Can you work these out from the drawing? Everything is in mm from the part's minimum corner. Give positions to 0.01 mm unless a question says otherwise; leave off trailing zeros. Write each loop counter-clockwise with the first axis right and the second up, starting at its lowest first coordinate (ties: lowest second). Pieces come first, ordered by that corner, then holes. Notation, with made-up numbers: (23, 18.5) - (74, 18.5) arc R17 cw to (74, 47.5) - close; hole circle Ø2 at (-17.5, 21). An arc over 180 degrees is marked (long way). Write each question's results on one line, items separated by ' | '. Start each with the question number.
Item 1: Suppose I cut it at D-D on x = 2.5. List the corners of the cut face in (y, z) for me, then the cut area to 3 significant figures.
Item 2: Please list where these lines run through material, in increasing order: line 1 along Y through (x, z) = (14.5, 14.25); line 2 along Y through (x, z) = (11.75, 12.25); line 3 along X through (y, z) = (20, 10.25).
Item 3: Will this pin go through, and if not, where does the flat tip stop? P1, Ø5, axis at x = 10, z = 9, coming from the -Y side.
Item 4: Suppose I cut it at C-C on z = 23.75. List the corners of the cut face in (x, y) for me, then the cut area to 3 significant figures.
Item 5: We'd pull the mould along Y, two halves only. Please class the marked faces 1, 2 and 3: +Y half, -Y half, draft (parallel to the pull), parting line (faces both ways), or undercut.
Item 6: Suppose I cut it at A-A on y = 14.5. List the corners of the cut face in (x, z) for me, then the cut area to 4 significant figures.
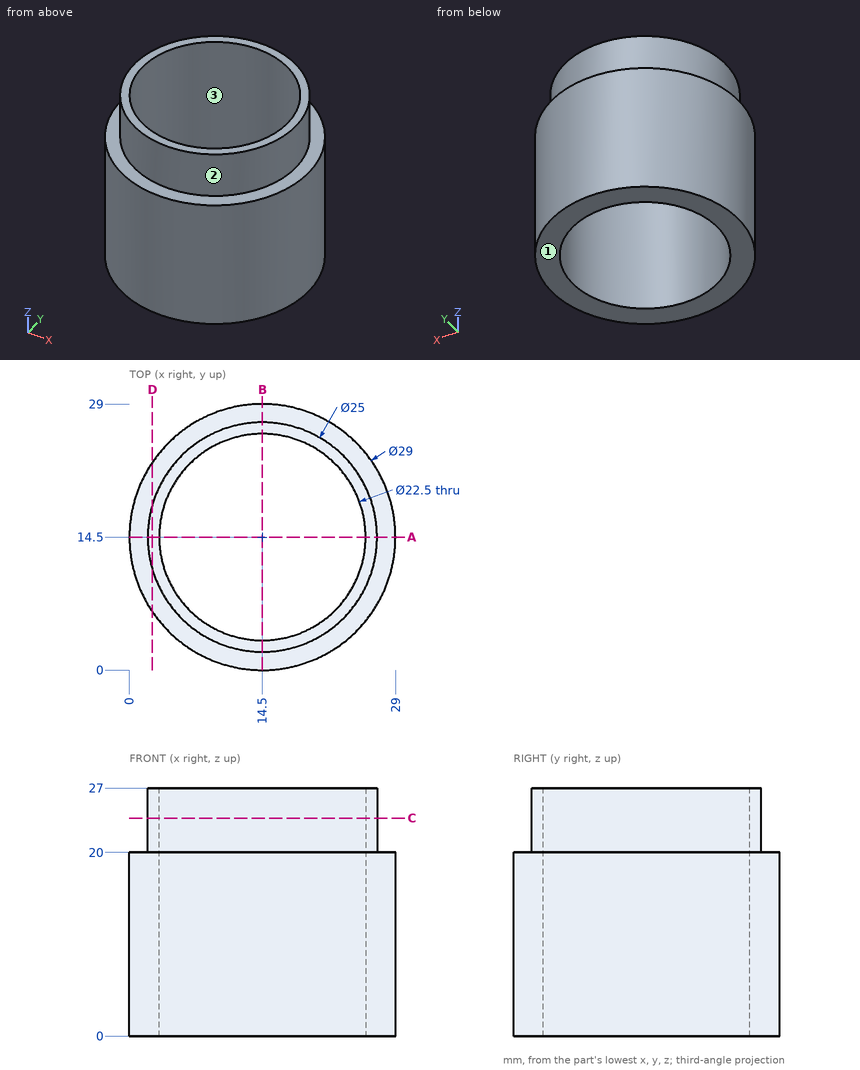
Checked values:
1) outline: (6.36, 0) - (22.64, 0) - (22.64, 20) - (18, 20) - (18, 27) - (11, 27) - (11, 20) - (6.36, 20) - close | area: 375 mm^2
2) line 1: y = 0 to 3.25, 25.75 to 29 | line 2: y = 0.26 to 3.59, 25.41 to 28.74 | line 3: x = 1.08 to 4.69, 24.31 to 27.92
3) P1: stops at y = 0.14
4) outline: circle Ø25 at (14.5, 14.5); hole circle Ø22.5 at (14.5, 14.5) | area: 93.3 mm^2
5) face 1: draft | face 2: parting line | face 3: undercut
6) outline: (0, 0) - (3.25, 0) - (3.25, 27) - (2, 27) - (2, 20) - (0, 20) - close; (25.75, 0) - (29, 0) - (29, 20) - (27, 20) - (27, 27) - (25.75, 27) - close | area: 147.5 mm^2
